```python
from build123d import *

# Parameters (mm, degrees)
SKETCH_1_W          = 9
SKETCH_1_H          = 40
EXTRUDE_1_DEPTH     = 6.3
SKETCH_2_W          = 9
SKETCH_2_H          = 25.5
EXTRUDE_2_DEPTH     = 5.3
SKETCH_3_R          = 1.65
CUT_EXTRUDE_1_DEPTH = 15.3
SKETCH_4_W          = 0.410265385
SKETCH_4_H          = 1.299173718
EXTRUDE_3_DEPTH     = 5
SKETCH_5_W          = 3
SKETCH_5_H          = 22
CUT_EXTRUDE_2_DEPTH = 8


with BuildPart() as part:
    # 草图1 → 拉伸1 (new body)
    with BuildSketch(Plane.XY):
        Rectangle(SKETCH_1_W, SKETCH_1_H)
    extrude(amount=EXTRUDE_1_DEPTH)

    # 草图2 → 拉伸2 (add)
    with BuildSketch(Plane.XY.offset(6.3)):
        Rectangle(SKETCH_2_W, SKETCH_2_H)
    extrude(amount=EXTRUDE_2_DEPTH)

    # 草图3 → 切除-拉伸1 (cut)
    with BuildSketch(Plane.XY.offset(6.3)):
        with Locations((0, 16.25)):
            Circle(SKETCH_3_R)
        with Locations((0, -16.25)):
            Circle(SKETCH_3_R)
    extrude(amount=-CUT_EXTRUDE_1_DEPTH, mode=Mode.SUBTRACT)

    # 草图4 → 拉伸3 (add)
    with BuildSketch(Plane(origin=(0, 0, 0), x_dir=(-1, 0, 0), z_dir=(0, 0, -1))):
        with Locations((2.428938656, 10)):
            Rectangle(SKETCH_4_W, SKETCH_4_H)
        with Locations((-2.113574837, 10)):
            Rectangle(SKETCH_4_W, SKETCH_4_H)
        with Locations((2.428938656, 5)):
            Rectangle(SKETCH_4_W, SKETCH_4_H)
        with Locations((-2.113574837, 5)):
            Rectangle(SKETCH_4_W, SKETCH_4_H)
        with Locations((2.428938656, 0)):
            Rectangle(SKETCH_4_W, SKETCH_4_H)
        with Locations((-2.113574837, 0)):
            Rectangle(SKETCH_4_W, SKETCH_4_H)
        with Locations((-2.113574837, -5)):
            Rectangle(SKETCH_4_W, SKETCH_4_H)
        with Locations((2.428938656, -5)):
            Rectangle(SKETCH_4_W, SKETCH_4_H)
        with Locations((-2.113574837, -10)):
            Rectangle(SKETCH_4_W, SKETCH_4_H)
        with Locations((2.428938656, -10)):
            Rectangle(SKETCH_4_W, SKETCH_4_H)
    extrude(amount=EXTRUDE_3_DEPTH)

    # 草图5 → 切除-拉伸2 (cut)
    with BuildSketch(Plane.XY.offset(11.6)):
        Rectangle(SKETCH_5_W, SKETCH_5_H)
    extrude(amount=-CUT_EXTRUDE_2_DEPTH, mode=Mode.SUBTRACT)


solid = part.part
```
Could you check a few things on this model? Use its own coordinates, in mm. A direction names the side the tool comes from. Give positions to 0.01 mm unless a question says otherwise; leave off trailing zeros. Loops run counter-clockwise (first coordinate to the right, second up) from the corner with the lowest first, then second, coordinate; pieces in that order, holes last. Notation, with made-up numbers: (37.25, 71) -> (70.25, 71) arc R22 cw to (70.25, 101) -> close; hole circle Ø4 at (19, 8). An arc over 180 degrees is marked (long way). Put each result on its own line as item: value.
(1) Imagine slicing it at D-D on y = 8. Write out the boundary of the cut face in (x, z).
Computed:
outline: (-4.5, 0) -> (4.5, 0) -> (4.5, 11.6) -> (1.5, 11.6) -> (1.5, 3.6) -> (-1.5, 3.6) -> (-1.5, 11.6) -> (-4.5, 11.6) -> close
(2) Imagine slicing it at B-B on y = 16.25. Write out the boundary of the cut face in (x, z).
Computed:
outline: (-4.5, 0) -> (-1.65, 0) -> (-1.65, 6.3) -> (-4.5, 6.3) -> close; (1.65, 0) -> (4.5, 0) -> (4.5, 6.3) -> (1.65, 6.3) -> close
(3) I'm going to push flat-ended pins straight in: pin 1 Ø1 at (y, z) = (-0.5, -2) entering from -X; pin 2 Ø1 at (x, z) = (-3, -3.5) entering from +Y; pin 3 Ø3.5 at (x, y) = (-1, -17.5) entering from +Z. Where does each tip first touch, or does it pass through?
Computed:
pin 1: x = -2.63
pin 2: y = 10.65
pin 3: z = 6.3
(4) Please list where these lines run through material, in increasing order: probe 1 along Y at (x, z) = (-2.5, -2); probe 2 along Y at (x, z) = (0, 2.25); probe 3 along Y at (x, z) = (0, 3.75). Write a range as [from, to].
Computed:
probe 1: [-10.65, -9.35], [-5.65, -4.35], [-0.65, 0.65], [4.35, 5.65], [9.35, 10.65]
probe 2: [-20, -17.9], [-14.6, 14.6], [17.9, 20]
probe 3: [-20, -17.9], [-14.6, -11], [11, 14.6], [17.9, 20]
(5) Imagine slicing it at A-A on x = 0. Write out the boundary of the cut face in (y, z).
Computed:
outline: (-20, 0) -> (-17.9, 0) -> (-17.9, 6.3) -> (-20, 6.3) -> close; (-14.6, 0) -> (14.6, 0) -> (14.6, 6.3) -> (12.75, 6.3) -> (12.75, 11.6) -> (11, 11.6) -> (11, 3.6) -> (-11, 3.6) -> (-11, 11.6) -> (-12.75, 11.6) -> (-12.75, 6.3) -> (-14.6, 6.3) -> close; (17.9, 0) -> (20, 0) -> (20, 6.3) -> (17.9, 6.3) -> close
(6) Imagine slicing it at C-C on z = 7.5. Write out the boundary of the cut face in (x, y), plus the area to 4 significant figures.
Computed:
outline: (-4.5, -12.75) -> (4.5, -12.75) -> (4.5, 12.75) -> (-4.5, 12.75) -> close; hole (-1.5, -11) -> (1.5, -11) -> (1.5, 11) -> (-1.5, 11) -> close
area: 163.5 mm^2
(7) Thinking about a two-plate mould opening in Y: for faces 1 (the face through (0, -12.75, 9)), 2 (the face through (-4.5, 0, 4)), 3 (the face through (0, 11, 8)), which applies, pulls with the +Y half, pulls with the -Y half, needs draft (parallel to the pull), parting line crosses it, or undercut?
Computed:
face 1: pulls with the -Y half
face 2: needs draft
face 3: undercut
(8) For faces 4 (the face through (-1.5, 0, 8)), 5 (the face through (1.908, 0, -2)), 6 (the face through (-0.36, -17.86, 3.19)), 7 (the face through (2.319, 10, -2)), 8 (the face through (-1, -18, 6.3)), which set-ups out of +Z, -Z, +X, -X, +Y, -Y let a thin tool reach every point of the face, with its end or its side?
Computed:
face 4: +Z
face 5: -Z, +Y, -Y
face 6: +Z, -Z
face 7: -Z, +X, +Y, -Y
face 8: +Z, +X, -X, -Y
